from build123d import *

# Parameters (mm, degrees)
BASE_EXTRUDE_DEPTH = 838.2
CUT_EXTRUDE1_DEPTH = 38.1
SKETCH5_R          = 3.9751
CUT_EXTRUDE3_DEPTH = 827.640765765
SKETCH6_R          = 3.9751
CUT_EXTRUDE4_DEPTH = 827.640765765


with BuildPart() as part:
    # Sketch1 → Base-Extrude (new, symmetric)
    with BuildSketch(Plane.XY):
        with BuildLine():
            Line((-12.7, 38.1), (12.7, 38.1))
            ThreePointArc((12.7, 38.1), (21.680256121, 34.380256121), (25.4, 25.4))
            Line((25.4, 25.4), (25.4, -25.4))
            ThreePointArc((25.4, -25.4), (21.680256121, -34.380256121), (12.7, -38.1))
            Line((12.7, -38.1), (-12.7, -38.1))
            ThreePointArc((-12.7, -38.1), (-21.680256121, -34.380256121), (-25.4, -25.4))
            Line((-25.4, -25.4), (-25.4, 25.4))
            ThreePointArc((-25.4, 25.4), (-21.680256121, 34.380256121), (-12.7, 38.1))
        make_face()
        with BuildLine():
            Line((-20.6248, 25.4), (-20.6248, -25.4))
            ThreePointArc((-20.6248, -25.4), (-18.30367982, -31.00367982), (-12.7, -33.3248))
            Line((-12.7, -33.3248), (12.7, -33.3248))
            ThreePointArc((12.7, -33.3248), (18.30367982, -31.00367982), (20.6248, -25.4))
            Line((20.6248, -25.4), (20.6248, 25.4))
            ThreePointArc((20.6248, 25.4), (18.30367982, 31.00367982), (12.7, 33.3248))
            Line((12.7, 33.3248), (-12.7, 33.3248))
            ThreePointArc((-12.7, 33.3248), (-18.30367982, 31.00367982), (-20.6248, 25.4))
        make_face(mode=Mode.SUBTRACT)
    extrude(amount=BASE_EXTRUDE_DEPTH, both=True)

    # Sketch2 → Cut-Extrude1 (cut, symmetric)
    with BuildSketch(Plane(origin=(0, 0, 0), x_dir=(0, 0, -1), z_dir=(1, 0, 0))):
        Polygon((-811.795200446, 121.113483343), (-832.45021311, -121.113483343), (-857.85021311, -121.113483343), (-857.85021311, 121.113483343), align=None)
        Polygon((833.122276443, 128.994953344), (811.123137113, -128.994953344), (858.522276443, -128.994953344), (858.522276443, 128.994953344), align=None)
    extrude(amount=CUT_EXTRUDE1_DEPTH, both=True, mode=Mode.SUBTRACT)

    # Sketch5 → Cut-Extrude3 (cut, through all)
    with BuildSketch(Plane(origin=(0, 0, 0), x_dir=(1, 0, 0), z_dir=(0, 1, 0))):
        with Locations(Location((0, 806.45, 0), (0, 0, 270))):
            Circle(SKETCH5_R)
    extrude(amount=-CUT_EXTRUDE3_DEPTH, mode=Mode.SUBTRACT)

    # Sketch6 → Cut-Extrude4 (cut, through all)
    with BuildSketch(Plane(origin=(0, 0, 0), x_dir=(1, 0, 0), z_dir=(0, 1, 0))):
        with Locations(Location((0, 812.8, 0), (0, 0, 90))):
            Circle(SKETCH6_R)
    extrude(amount=CUT_EXTRUDE4_DEPTH, mode=Mode.SUBTRACT)


solid = part.part
Work out the finished part from the listing and answer in its coordinate system (mm). A direction names the side the tool comes from. Give positions to 0.01 mm unless a question says otherwise; leave off trailing zeros. Order: outer loops, then holes, each group sorted by start corner. A loop starts at its lowest first (then second) coordinate and runs counter-clockwise, first axis right, second up. Notation, with made-up numbers: (45.25, -36) - (60.25, -36) arc R21 cw to (60.25, -26) - close; hole circle Ø11 at (74, 76). An arc over 180 degrees is marked (long way). Answer as CSV lines item,"result". Start each with the question number.
Q1. Find the intervals of material crossed by L1, parallel to Y at x = -8.5, z = 588.5; L2, parallel to Y at x = -14, z = -160; L3, parallel to X at y = -23, z = -718.5, in increasing order. Write a range as [from, to].
Q2. The part is cut by section B-B (y = 6). Write down the section's boundary in (x, z), then the cut area to 3 significant figures.
Q3. For faces 1 (the face through (25.4, 0, 12)), 2 (the face through (0, -33.325, 14)), determine the directions among +Z, -Z, +X, -X, +Y, -Y from which every point of the face is accessible in a straight line to the end or side of a thin tool.
Q4. Given pin 1 Ø7 at (x, z) = (0, -812.8) entering from +Y, flat-ended and moving along its own axis, determine where the tip first touches the part or whether it passes through.
Q5. The part is cut by section A-A (z = -198). Write down the section's boundary in (x, y).
Check result:
1,L1,"y = [-38.1, -33.32], [33.32, 38.1]"
1,L2,"y = [-38.03, -33.22], [33.22, 38.03]"
1,L3,"x = [-25.4, -20.62], [20.62, 25.4]"
2,outline,"(-25.4, -822.63) - (-20.62, -822.63) - (-20.62, 821.61) - (-25.4, 821.61) - close; (20.62, -822.63) - (25.4, -822.63) - (25.4, 821.61) - (20.62, 821.61) - close"
2,area,"15,700 mm²"
3,face 1,"+Z, -Z, +X, +Y, -Y"
3,face 2,"+Z, -Z"
4,pin 1,"stops at y = -33.32"
5,outline,"(-25.4, -25.4) arc R12.7 ccw to (-12.7, -38.1) - (12.7, -38.1) arc R12.7 ccw to (25.4, -25.4) - (25.4, 25.4) arc R12.7 ccw to (12.7, 38.1) - (-12.7, 38.1) arc R12.7 ccw to (-25.4, 25.4) - close; hole (-20.62, -25.4) arc R7.92 ccw to (-12.7, -33.32) - (12.7, -33.32) arc R7.92 ccw to (20.62, -25.4) - (20.62, 25.4) arc R7.92 ccw to (12.7, 33.32) - (-12.7, 33.32) arc R7.92 ccw to (-20.62, 25.4) - close"
